Answer from the drawing. Dimensions are ordinates in mm from the lowest x, y and z of the part. Give positions to 0.01 mm unless a question says otherwise; leave off trailing zeros. Write each loop counter-clockwise with the first axis right and the second up, starting at its lowest first coordinate (ties: lowest second). Pieces come first, ordered by that corner, then holes.
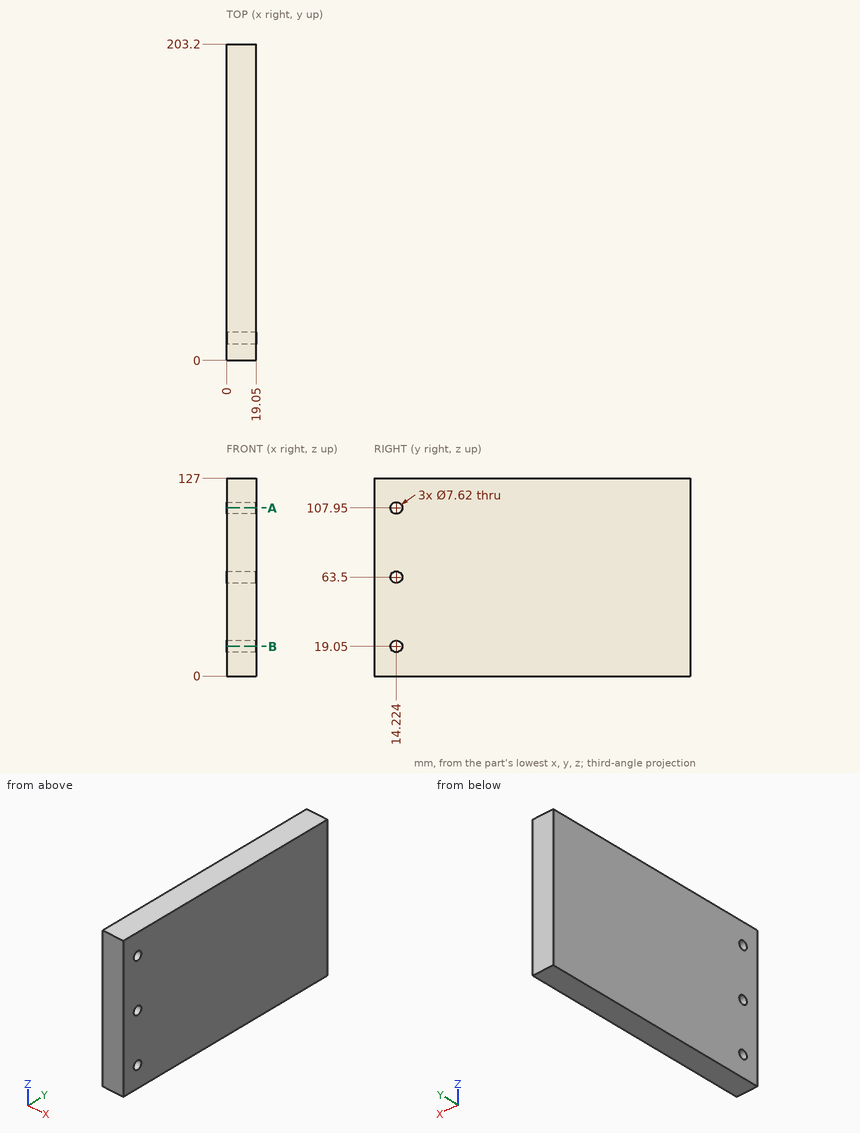
Item 1: Section A-A (z = 107.95) is taken. Write down the section's boundary in (x, y).
Result set:
outline: (0, 0) - (19.05, 0) - (19.05, 10.41) - (0, 10.41) - close; (0, 18.03) - (19.05, 18.03) - (19.05, 203.2) - (0, 203.2) - close
Item 2: This flat-tipped pin is pushed along its axis until it touches: pin 1 Ø4.5 at (y, z) = (14.224, 19.05) entering from -X. Where does it stop, or does it pass through?
Result set:
pin 1: passes through
Item 3: Find the intervals of material crossed by line 1 along Y through (x, z) = (5, 19.05); line 2 along Y through (x, z) = (8, 17.5), in increasing order.
Result set:
line 1: y = 0 to 10.41, 18.03 to 203.2
line 2: y = 0 to 10.74, 17.7 to 203.2
